Read the model definition and answer for the solid it produces. Units are mm, in the model's axes. A direction names the side the tool comes from. Coordinates: 2 decimals unless noted, no trailing zeros. Order: outer loops, then holes, each group sorted by start corner. A loop starts at its lowest first (then second) coordinate and runs counter-clockwise, first axis right, second up. Notation, with made-up numbers: (-24.5, 50.5) -> (3.5, 50.5) arc R15 ccw to (3.5, 64.5) -> close; hole circle Ø3 at (79.25, -30.5). An arc over 180 degrees is marked (long way). Answer as a JSON object with one key per item and string values. Group by question number.
1) Section A-A on x = 0 is taken. Determine the outline of the cut face in (y, z).
2) Section D-D on y = -25 is taken. Determine the outline of the cut face in (x, z), and give its area (3 significant figures).
3) Section C-C on x = 100 is taken. Determine the outline of the cut face in (y, z).
4) Given pin 1 (13 mm diameter, centred on x = -125, y = -25, fed in from -Z); pin 2 (6.5 mm diameter, centred on x = -62.5, y = -25, fed in from +Z); pin 3 (13 mm diameter, centred on x = 0, y = -13, fed in from +Z), each flat-ended and moving along its own axis, determine where each tip first touches the part or whether it passes through.
5) Consider L1, parallel to Y at x = 125, z = 5.75; L2, parallel to X at y = 24.5, z = 5.5; L3, parallel to Y at x = -100, z = 2.5. Determine where each line is inside the solid, lowest interval first.
6) A tool of negligible diameter and unlimited length cuts with its end or side. For faces 1 (the cylindrical face through (80.02, -0.88, -1.01)), 2 (the cylindrical face through (4, -19, 3)), 3 (the flat face through (-2, 35, 3)), from which of +Z, -Z, +X, -X, +Y, -Y can it reach the whole face along a straight path? Write none if from no direction.
7) Section B-B on z = 5.25 is taken. Count the separate pieces of the cut face and the enclosed holes in it, and give its area (3 significant figures).
8) Determine the mould class of faces 4 (the cylindrical face through (133.289, 33.196, 3.549)), 5 (the cylindrical face through (-133.289, 33.196, 3.549)), 6 (the cylindrical face through (-4, -19, 3)), 7 (the flat face through (103, -15, -2)) for opening direction X: released by +X, released by -X, zero draft, split by the parting line, or undercut.
from build123d import *

# Parameters (mm, degrees)
SKETCH1_W           = 270
SKETCH1_H           = 70
BOSS_EXTRUDE1_DEPTH = 7
FILLET1_R           = 6
SKETCH2_R           = 15
SKETCH2_R_2         = 4
CUT_EXTRUDE1_DEPTH  = 10
BOSS_EXTRUDE2_START = 2
SKETCH3_R           = 20
SKETCH3_R_2         = 15
BOSS_EXTRUDE2_DEPTH = 2


with BuildPart() as part:
    # Sketch1 → Boss-Extrude1 (new body)
    with BuildSketch(Plane.XY):
        Rectangle(SKETCH1_W, SKETCH1_H)
    extrude(amount=BOSS_EXTRUDE1_DEPTH)

    # Fillet1
    fillet1_edges = [part.edges().sort_by_distance(p)[0] for p in [
        (135, -35, 3.5),
        (-135, -35, 3.5),
        (-135, 35, 3.5),
        (135, 35, 3.5),
    ]]
    fillet(fillet1_edges, radius=FILLET1_R)

    # Sketch2 → Cut-Extrude1 (cut)
    with BuildSketch(Plane(origin=(0, 0, 0), x_dir=(-1, 0, 0), z_dir=(0, 0, -1))):
        with Locations((-100, 0)):
            Circle(SKETCH2_R)
        with Locations((100, 0)):
            Circle(SKETCH2_R)
        with Locations((125, 25)):
            Circle(SKETCH2_R_2)
        with Locations((62.5, 25)):
            Circle(SKETCH2_R_2)
        with Locations((-62.5, 25)):
            Circle(SKETCH2_R_2)
        with Locations((-125, 25)):
            Circle(SKETCH2_R_2)
        with Locations(Location((-125, -25, 0), (0, 0, 180))):
            Circle(SKETCH2_R_2)
        with Locations(Location((-62.5, -25, 0), (0, 0, 180))):
            Circle(SKETCH2_R_2)
        with Locations(Location((62.5, -25, 0), (0, 0, 180))):
            Circle(SKETCH2_R_2)
        with Locations(Location((125, -25, 0), (0, 0, 180))):
            Circle(SKETCH2_R_2)
        with BuildLine():
            ThreePointArc((2.645751311, 22), (0, 29), (-2.645751311, 22))
            ThreePointArc((-2.645751311, 22), (-4, 19), (-2.645751311, 16))
            ThreePointArc((-2.645751311, 16), (0, 9), (2.645751311, 16))
            ThreePointArc((2.645751311, 16), (4, 19), (2.645751311, 22))
        make_face()
        with BuildLine():
            ThreePointArc((2.645751311, -22), (0, -29), (-2.645751311, -22))
            ThreePointArc((-2.645751311, -22), (-4, -19), (-2.645751311, -16))
            ThreePointArc((-2.645751311, -16), (0, -9), (2.645751311, -16))
            ThreePointArc((2.645751311, -16), (4, -19), (2.645751311, -22))
        make_face()
    extrude(amount=-CUT_EXTRUDE1_DEPTH, mode=Mode.SUBTRACT)

    # Sketch3 → Boss-Extrude2 (add)
    # profile 1 of 2: a face of its own
    with BuildSketch(Plane(origin=(0, 0, 0), x_dir=(-1, 0, 0), z_dir=(0, 0, -1)).offset(BOSS_EXTRUDE2_START)):
        with Locations(Location((-100, 0, 0), (0, 0, 180))):
            Circle(SKETCH3_R)
        with Locations((-100, 0)):
            Circle(SKETCH3_R_2, mode=Mode.SUBTRACT)
    # profile 2 of 2: a face of its own
    with BuildSketch(Plane(origin=(0, 0, 0), x_dir=(-1, 0, 0), z_dir=(0, 0, -1)).offset(BOSS_EXTRUDE2_START)):
        with Locations(Location((100, 0, 0), (0, 0, 180))):
            Circle(SKETCH3_R)
        with Locations((100, 0)):
            Circle(SKETCH3_R_2, mode=Mode.SUBTRACT)
    extrude(amount=-BOSS_EXTRUDE2_DEPTH)


solid = part.part
Worked answers:
{
 "1": {"outline": "(-35, 0) -> (-29, 0) -> (-29, 7) -> (-35, 7) -> close; (-9, 0) -> (9, 0) -> (9, 7) -> (-9, 7) -> close; (29, 0) -> (35, 0) -> (35, 7) -> (29, 7) -> close"},
 "2": {"outline": "(-135, 0) -> (-129, 0) -> (-129, 7) -> (-135, 7) -> close; (-121, 0) -> (-66.5, 0) -> (-66.5, 7) -> (-121, 7) -> close; (-58.5, 0) -> (-4, 0) -> (-4, 7) -> (-58.5, 7) -> close; (4, 0) -> (58.5, 0) -> (58.5, 7) -> (4, 7) -> close; (66.5, 0) -> (121, 0) -> (121, 7) -> (66.5, 7) -> close; (129, 0) -> (135, 0) -> (135, 7) -> (129, 7) -> close", "area": "1,610 mm²"},
 "3": {"outline": "(-35, 0) -> (-20, 0) -> (-20, -2) -> (-15, -2) -> (-15, 7) -> (-35, 7) -> close; (15, -2) -> (20, -2) -> (20, 0) -> (35, 0) -> (35, 7) -> (15, 7) -> close"},
 "4": {"pin 1": "stops at z = 0", "pin 2": "passes through", "pin 3": "stops at z = 7"},
 "5": {"L1": "y = -35 to -29, -21 to 21, 29 to 35", "L2": "x = -135 to -128.97, -121.03 to -66.47, -58.53 to -3.97, 3.97 to 58.53, 66.47 to 121.03, 128.97 to 135", "L3": "y = -35 to -15, 15 to 35"},
 "6": {"face 1": "-Z", "face 2": "+Z, -Z", "face 3": "+Z, -Z, +X, -X, +Y"},
 "7": {"separate pieces": "1", "enclosed holes": "12", "area": "16,800 mm²"},
 "8": {"face 4": "released by +X", "face 5": "released by -X", "face 6": "undercut", "face 7": "zero draft"}
}
